Verification items for the finished model (mm, model axes). A direction names the side the tool comes from. Coordinates: 2 decimals unless noted, no trailing zeros. Write each loop counter-clockwise with the first axis right and the second up, starting at its lowest first coordinate (ties: lowest second). Pieces come first, ordered by that corner, then holes. Notation, with made-up numbers: (37.25, 87) -> (65.25, 87) arc R16 cw to (65.25, 113) -> close; hole circle Ø7 at (12, 54). An arc over 180 degrees is marked (long way). Write item = value, one per line. Start each with the question number.
(1) Section check C-C (z = 156). Record the cut outline in (x, y), plus the area to 3 significant figures.
(2) Gauge pin test, flat ends, axial feed: pin 1 Ø4.5 at (x, z) = (60, 156) entering from +Y; pin 2 Ø2 at (y, z) = (48, 152) entering from -X; pin 3 Ø1.2 at (x, z) = (22.5, 141) entering from +Y. Record the tip position at first contact, or that the pin passes through.
(3) Set-up check for faces 1 (the face through (26, 72, 142)), 2 (the face through (76, 21, 142)), 3 (the face through (50, 76, 142)): record each of +Z, -Z, +X, -X, +Y, -Y from which the full face is reachable in a straight line by a thin tool's end or side.
(4) Material ranges on probe 1 along Y at (x, z) = (35, 141.25); probe 2 along Y at (x, z) = (85, 141.3); probe 3 along Z at (x, y) = (60, 38.8), recorded low to high. Write a range as [from, to].
(5) Section check B-B (x = 56). Record the cut outline in (y, z).
(6) Mould release check, pull along Y, two halves, no side actions. Record for faces 4 (the face through (76, 84, 142)), 5 (the face through (81, 43, 144)), 6 (the face through (48, 62, 142)), 7 (the face through (72.92, 78.86, 141.97)): released by +Y, released by -Y, zero draft, split by the parting line, or undercut.
(7) Section check D-D (y = 60.5). Record the cut outline in (x, z), plus the area to 3 significant figures.
(8) Section check A-A (y = 10). Record the cut outline in (x, z), plus the area to 3 significant figures.
```python
from build123d import *

# Parameters (mm, degrees)
CYLINDER_R             = 2
CYLINDER_DEPTH         = 50
BOX083_W               = 24
BOX083_H               = 13
BOX083_DEPTH           = 10
BOX082_W               = 40
BOX082_H               = 17
BOX082_DEPTH           = 10
BOX081_W               = 25
BOX081_H               = 36
BOX081_DEPTH           = 10
BOX084_W               = 24
BOX084_H               = 13
BOX084_DEPTH           = 10
BOX080_W               = 25
BOX080_H               = 36
BOX080_DEPTH           = 10
BOX085_W               = 15
BOX085_H               = 20
BOX085_DEPTH           = 10
BOX073_W               = 18
BOX073_H               = 10
BOX073_DEPTH           = 25
BOX086_W               = 28
BOX086_H               = 22
BOX086_DEPTH           = 25
CYLINDER107_R          = 1
CYLINDER107_DEPTH      = 10
CYLINDER103_R          = 2.25
CYLINDER103_DEPTH      = 10
CYLINDER104_R          = 2.25
CYLINDER104_DEPTH      = 10
CYLINDER106_R          = 2
CYLINDER106_DEPTH      = 10
CYLINDER105_R          = 2.25
CYLINDER105_DEPTH      = 10
BOX063_W               = 26
BOX063_H               = 12
BOX063_DEPTH           = 4
BOX061_W               = 26
BOX061_H               = 12
BOX061_DEPTH           = 4
BOX062_W               = 26
BOX062_H               = 12
BOX062_DEPTH           = 4
BOX064_W               = 26
BOX064_H               = 12
BOX064_DEPTH           = 4
BOX060_W               = 94
BOX060_H               = 80
BOX060_DEPTH           = 4
CUT020_PLACEMENT_ANGLE = 180


with BuildPart() as cylinder:
    # Cylinder → Cylinder (new body)
    with BuildSketch(Plane(origin=(60, 17, 156), x_dir=(1, 0, 0), z_dir=(0, 1, 0))):
        Circle(CYLINDER_R)
    extrude(amount=CYLINDER_DEPTH)


with BuildPart() as cube041:
    # Box083 → Box083 (new body)
    with BuildSketch(Plane(origin=(48, 21, 140), x_dir=(1, 0, 0), z_dir=(0, 0, 1))):
        with Locations((12, 6.5)):
            Rectangle(BOX083_W, BOX083_H)
    extrude(amount=BOX083_DEPTH)


with BuildPart() as cube040:
    # Box082 → Box082 (new body)
    with BuildSketch(Plane(origin=(40, 4, 140), x_dir=(1, 0, 0), z_dir=(0, 0, 1))):
        with Locations((20, 8.5)):
            Rectangle(BOX082_W, BOX082_H)
    extrude(amount=BOX082_DEPTH)


with BuildPart() as cube039:
    # Box081 → Box081 (new body)
    with BuildSketch(Plane(origin=(82, 26, 140), x_dir=(1, 0, 0), z_dir=(0, 0, 1))):
        with Locations((12.5, 18)):
            Rectangle(BOX081_W, BOX081_H)
    extrude(amount=BOX081_DEPTH)


with BuildPart() as cube042:
    # Box084 → Box084 (new body)
    with BuildSketch(Plane(origin=(48, 56, 140), x_dir=(1, 0, 0), z_dir=(0, 0, 1))):
        with Locations((12, 6.5)):
            Rectangle(BOX084_W, BOX084_H)
    extrude(amount=BOX084_DEPTH)


with BuildPart() as cube038:
    # Box080 → Box080 (new body)
    with BuildSketch(Plane(origin=(13, 26, 140), x_dir=(1, 0, 0), z_dir=(0, 0, 1))):
        with Locations((12.5, 18)):
            Rectangle(BOX080_W, BOX080_H)
    extrude(amount=BOX080_DEPTH)


with BuildPart() as basecuts:
    # Box085 → Box085 (new body)
    with BuildSketch(Plane(origin=(70, 69, 140), x_dir=(0, 1, 0), z_dir=(0, 0, 1))):
        with Locations((7.5, 10)):
            Rectangle(BOX085_W, BOX085_H)
    extrude(amount=BOX085_DEPTH)

    # Fusion133: union Cube041, Cube040, Cube039, Cube042, Cube038
    add(cube041.part)
    add(cube040.part)
    add(cube039.part)
    add(cube042.part)
    add(cube038.part)


with BuildPart() as basecuts001:
    # Box073 → Box073 (new body)
    with BuildSketch(Plane(origin=(51, 40, 140), x_dir=(1, 0, 0), z_dir=(0, 0, 1))):
        with Locations((9, 5)):
            Rectangle(BOX073_W, BOX073_H)
    extrude(amount=BOX073_DEPTH)

    # Fusion134: union baseCuts
    add(basecuts.part)


with BuildPart() as obj1:
    # Box086 → Box086 (new body)
    with BuildSketch(Plane(origin=(46, 34, 140), x_dir=(1, 0, 0), z_dir=(0, 0, 1))):
        with Locations((14, 11)):
            Rectangle(BOX086_W, BOX086_H)
    extrude(amount=BOX086_DEPTH)


with BuildPart() as cylinder109:
    # Cylinder107 → Cylinder107 (new body)
    with BuildSketch(Plane.XY):
        Circle(CYLINDER107_R)
    extrude(amount=CYLINDER107_DEPTH)


with BuildPart() as cylinder107:
    # Cylinder103 → Cylinder103 (new body)
    with BuildSketch(Plane(origin=(62, 3, 0), x_dir=(1, 0, 0), z_dir=(0, 0, 1))):
        Circle(CYLINDER103_R)
    extrude(amount=CYLINDER103_DEPTH)


with BuildPart() as cylinder103:
    # Cylinder104 → Cylinder104 (new body)
    with BuildSketch(Plane(origin=(72, 71, 0), x_dir=(1, 0, 0), z_dir=(0, 0, 1))):
        Circle(CYLINDER104_R)
    extrude(amount=CYLINDER104_DEPTH)


with BuildPart() as cylinder104:
    # Cylinder106 → Cylinder106 (new body)
    with BuildSketch(Plane(origin=(22, 71, 0), x_dir=(1, 0, 0), z_dir=(0, 0, 1))):
        Circle(CYLINDER106_R)
    extrude(amount=CYLINDER106_DEPTH)


with BuildPart() as screwins001:
    # Cylinder105 → Cylinder105 (new body)
    with BuildSketch(Plane(origin=(32, 3, 0), x_dir=(1, 0, 0), z_dir=(0, 0, 1))):
        Circle(CYLINDER105_R)
    extrude(amount=CYLINDER105_DEPTH)

    # Fusion123: union Cylinder109, Cylinder107, Cylinder103, Cylinder104
    add(cylinder109.part)
    add(cylinder107.part)
    add(cylinder103.part)
    add(cylinder104.part)


with BuildPart() as screwins001_1:
    # Fusion123 placement: moved
    add(screwins001.part.moved(Location((0, 3, 0))))


with BuildPart() as base004:
    # Box063 → Box063 (new body)
    with BuildSketch(Plane(origin=(78, 68, 0), x_dir=(1, 0, 0), z_dir=(0, 0, 1))):
        with Locations((13, 6)):
            Rectangle(BOX063_W, BOX063_H)
    extrude(amount=BOX063_DEPTH)


with BuildPart() as base002:
    # Box061 → Box061 (new body)
    with BuildSketch(Plane.XY):
        with Locations((13, 6)):
            Rectangle(BOX061_W, BOX061_H)
    extrude(amount=BOX061_DEPTH)


with BuildPart() as base003:
    # Box062 → Box062 (new body)
    with BuildSketch(Plane(origin=(68, 0, 0), x_dir=(1, 0, 0), z_dir=(0, 0, 1))):
        with Locations((13, 6)):
            Rectangle(BOX062_W, BOX062_H)
    extrude(amount=BOX062_DEPTH)


with BuildPart() as fusion122:
    # Box064 → Box064 (new body)
    with BuildSketch(Plane(origin=(-10.25, 68, 0), x_dir=(1, 0, 0), z_dir=(0, 0, 1))):
        with Locations((13, 6)):
            Rectangle(BOX064_W, BOX064_H)
    extrude(amount=BOX064_DEPTH)

    # Fusion122: union base004, base002, base003
    add(base004.part)
    add(base002.part)
    add(base003.part)


with BuildPart() as spine:
    # Box060 → Box060 (new body)
    with BuildSketch(Plane.XY):
        with Locations((47, 40)):
            Rectangle(BOX060_W, BOX060_H)
    extrude(amount=BOX060_DEPTH)

    # Cut019: cut Fusion122
    add(fusion122.part, mode=Mode.SUBTRACT)

    # Cut020: cut screwIns001
    add(screwins001_1.part, mode=Mode.SUBTRACT)


with BuildPart() as spine_1:
    # Cut020 placement: moved
    add(spine.part.moved(Location((107, 84, 140))).rotate(Axis((107, 84, 140), (0, 0, 1)), CUT020_PLACEMENT_ANGLE))

    # Fusion: union obj1
    add(obj1.part)

    # Cut: cut baseCuts001
    add(basecuts001.part, mode=Mode.SUBTRACT)

    # Cut021: cut Cylinder
    add(cylinder.part, mode=Mode.SUBTRACT)


solid = spine_1.part
```
Response:
q1.outline = (46, 34) -> (58, 34) -> (58, 40) -> (51, 40) -> (51, 50) -> (58, 50) -> (58, 56) -> (46, 56) -> close; (62, 34) -> (74, 34) -> (74, 56) -> (62, 56) -> (62, 50) -> (69, 50) -> (69, 40) -> (62, 40) -> close
q1.area = 388 mm2
q2.pin_1 = 56
q2.pin_2 = 46
q2.pin_3 = 72
q3.face_1 = +Z, -Z, -X, +Y
q3.face_2 = +Z, -Z, -Y
q3.face_3 = +Z, -Z, +Y
q4.probe_1 = [4, 7.75], [12.25, 26], [62, 72]
q4.probe_2 = [4, 8], [12, 26], [62, 72]
q4.probe_3 = [140, 154], [158, 165]
q5.outline = (34, 140) -> (40, 140) -> (40, 165) -> (34, 165) -> close; (50, 140) -> (56, 140) -> (56, 165) -> (50, 165) -> close
q6.face_4 = released by +Y
q6.face_5 = zero draft
q6.face_6 = undercut
q6.face_7 = undercut
q7.outline = (38, 140) -> (48, 140) -> (48, 144) -> (38, 144) -> close; (72, 140) -> (82, 140) -> (82, 144) -> (72, 144) -> close
q7.area = 80.0 mm2
q8.outline = (29, 140) -> (32.75, 140) -> (32.75, 144) -> (29, 144) -> close; (37.25, 140) -> (40, 140) -> (40, 144) -> (37.25, 144) -> close; (80, 140) -> (83, 140) -> (83, 144) -> (80, 144) -> close; (87, 140) -> (91.25, 140) -> (91.25, 144) -> (87, 144) -> close
q8.area = 55.0 mm2
